Part model, mm, in its own coordinate system. Face numbers are marked on the shaded views. Give positions to 0.01 mm unless a question says otherwise; leave off trailing zeros. Order: outer loops, then holes, each group sorted by start corner. A loop starts at its lowest first (then second) coordinate and runs counter-clockwise, first axis right, second up. Notation, with made-up numbers: (-30, 23) - (-11, 23) arc R22 cw to (-11, 42) - close; hole circle Ø6 at (-33, 19.25). An arc over 180 degrees is marked (long way). One line per item, written item: value.
```python
from build123d import *

# Parameters (mm, degrees)
MOLD_BLOCK_WITH_RIDGES_DEPTH  = 169
SKETCH2_W                     = 29
SKETCH2_H                     = 19
BOTTOM_LEDGE_DEPTH            = 10
ROD_ALIGNMENT_HOLE_DEPTH      = 2
ROD_ALIGNMENT_HOLE_DEPTH_BACK = 6
SUBTRACT_ACTUATOR_DEPTH       = 169


# Read off the part's stored shape, not the designer's step: subtract actuator
with BuildPart() as part:
    # Sketch1 → mold block with ridges (new body)
    with BuildSketch(Plane(origin=(0, 0, 0), x_dir=(1, 0, 0), z_dir=(0, 1, 0))):
        Polygon((3, 0), (26, 0), (26, -3), (29, -3), (29, 2.5), (29, 12.5), (0, 12.5), (0, 0), (0, -3), (3, -3), align=None)
    extrude(amount=MOLD_BLOCK_WITH_RIDGES_DEPTH)

    # Sketch2 → bottom ledge (add)
    with BuildSketch(Plane.XZ):
        with Locations((14.5, -3)):
            Rectangle(SKETCH2_W, SKETCH2_H)
    extrude(amount=BOTTOM_LEDGE_DEPTH)

    # Sketch3 → rod alignment hole (cut, two sides: drawn at the far end of the back side and taken through both)
    with BuildSketch(Plane(origin=(0, 0, 0), x_dir=(1, 0, 0), z_dir=(0, 1, 0)).offset(-ROD_ALIGNMENT_HOLE_DEPTH_BACK)):
        with BuildLine():
            Line((8.05077524, -0.1), (20.94922476, -0.1))
            ThreePointArc((20.94922476, -0.1), (14.5, 6.45), (8.05077524, -0.1))
        make_face()
    extrude(amount=ROD_ALIGNMENT_HOLE_DEPTH + ROD_ALIGNMENT_HOLE_DEPTH_BACK, mode=Mode.SUBTRACT)

    # subtract actuator outline → subtract actuator (cut)
    with BuildSketch(Plane(origin=(0, 0, 0), x_dir=(1, 0, 0), z_dir=(0, 1, 0))):
        with BuildLine():
            ThreePointArc((23.85, 0), (14.5, 9.35), (5.15, 0))
            Line((5.15, 0), (23.85, 0))
        make_face()
    extrude(amount=SUBTRACT_ACTUATOR_DEPTH, mode=Mode.SUBTRACT)


solid = part.part
```
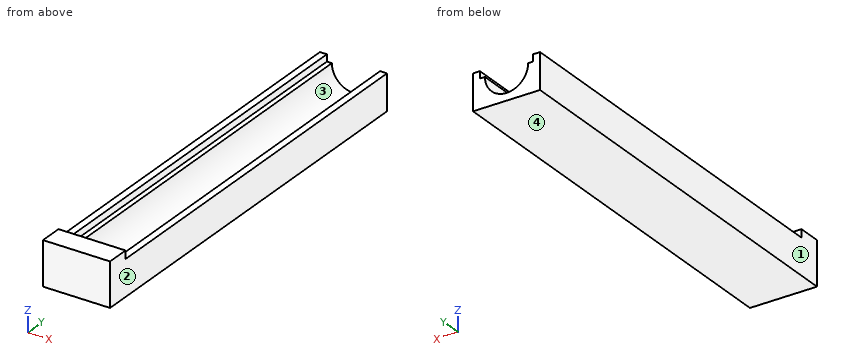
1) Two-plate mould, pull along X, no slides. Class the marked faces 1, 2, 3 and 4: pulls with the +X half, pulls with the -X half, needs draft (parallel to the pull), parting line crosses it, or undercut.
Answer:
face 1: pulls with the -X half
face 2: pulls with the +X half
face 3: undercut
face 4: needs draft
2) Slice it at A-A on x = 14.5. Write the cut outline in (y, z).
Answer:
outline: (-10, -12.5) - (169, -12.5) - (169, -9.35) - (0, -9.35) - (0, -6.45) - (-6, -6.45) - (-6, 0.1) - (0, 0.1) - (0, 6.5) - (-10, 6.5) - close
3) Drop flat-ended pins along their axis: P1, Ø1.5, axis at x = 27.5, y = 50, coming from the +Z side; P2, Ø5, axis at x = 15, y = 110, coming from the +Z side; P3, Ø7, axis at x = 16, z = -4.5, coming from the +Y side. Give the stop position or say it passes through.
Answer:
P1: stops at z = 3
P2: stops at z = -8.86
P3: stops at y = 0
4) Slice it at C-C on z = -3.75. Write the cut outline in (x, y).
Answer:
outline: (0, -10) - (29, -10) - (29, 169) - (23.07, 169) - (23.07, 0) - (19.75, 0) - (19.75, -6) - (9.25, -6) - (9.25, 0) - (5.93, 0) - (5.93, 169) - (0, 169) - close
5) Slice it at B-B on y = 99.5. Write the cut outline in (x, z), then the cut area to 3 significant figures.
Answer:
outline: (0, -12.5) - (29, -12.5) - (29, 3) - (26, 3) - (26, 0) - (23.85, 0) arc R9.35 cw to (5.15, 0) - (3, 0) - (3, 3) - (0, 3) - close
area: 243 mm2
6) Wall check: line 1 along X through (y, z) = (6.5, 2); line 2 along Y through (x, z) = (8, 5.25); line 3 along X through (y, z) = (141.5, -3). Give the ranges that are in metal, low to high. Write a range as [from, to].
Answer:
line 1: x = [0, 3], [26, 29]
line 2: y = [-10, 0]
line 3: x = [0, 5.64], [23.36, 29]
